from build123d import *

# Parameters (mm, degrees)
SKETCH1_R           = 27.5
BOSS_EXTRUDE1_DEPTH = 12


with BuildPart() as part:
    # Sketch1 → Boss-Extrude1 (new body)
    with BuildSketch(Plane.XY):
        Circle(SKETCH1_R)
        with BuildLine():
            Line((-3.977272727, 12.900825619), (-3.977272727, 17.042045114))
            ThreePointArc((-3.977272727, 17.042045114), (0, 17.5), (3.977272727, 17.042045114))
            Line((3.977272727, 17.042045114), (3.977272727, 12.900825619))
            ThreePointArc((3.977272727, 12.900825619), (6.75, 11.691342951), (9.183806352, 9.894832029))
            Line((9.183806352, 9.894832029), (12.770207637, 11.965441776))
            ThreePointArc((12.770207637, 11.965441776), (15.155444566, 8.75), (16.747480364, 5.076603337))
            Line((16.747480364, 5.076603337), (13.16107908, 3.00599359))
            ThreePointArc((13.16107908, 3.00599359), (13.5, 0), (13.16107908, -3.00599359))
            Line((13.16107908, -3.00599359), (16.747480364, -5.076603337))
            ThreePointArc((16.747480364, -5.076603337), (15.155444566, -8.75), (12.770207637, -11.965441776))
            Line((12.770207637, -11.965441776), (9.183806352, -9.894832029))
            ThreePointArc((9.183806352, -9.894832029), (6.75, -11.691342951), (3.977272727, -12.900825619))
            Line((3.977272727, -12.900825619), (3.977272727, -17.042045114))
            ThreePointArc((3.977272727, -17.042045114), (0, -17.5), (-3.977272727, -17.042045114))
            Line((-3.977272727, -17.042045114), (-3.977272727, -12.900825619))
            ThreePointArc((-3.977272727, -12.900825619), (-6.75, -11.691342951), (-9.183806352, -9.894832029))
            Line((-9.183806352, -9.894832029), (-12.770207637, -11.965441776))
            ThreePointArc((-12.770207637, -11.965441776), (-15.155444566, -8.75), (-16.747480364, -5.076603337))
            Line((-16.747480364, -5.076603337), (-13.16107908, -3.00599359))
            ThreePointArc((-13.16107908, -3.00599359), (-13.5, 0), (-13.16107908, 3.00599359))
            Line((-13.16107908, 3.00599359), (-16.747480364, 5.076603337))
            ThreePointArc((-16.747480364, 5.076603337), (-15.155444566, 8.75), (-12.770207637, 11.965441776))
            Line((-12.770207637, 11.965441776), (-9.183806352, 9.894832029))
            ThreePointArc((-9.183806352, 9.894832029), (-6.75, 11.691342951), (-3.977272727, 12.900825619))
        make_face(mode=Mode.SUBTRACT)
    extrude(amount=BOSS_EXTRUDE1_DEPTH)


solid = part.part
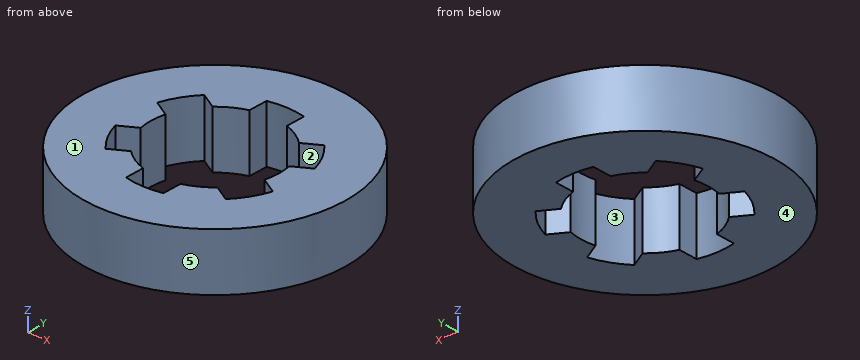
Geometry check sheet. Reference: the model listing, model coordinates, mm. Face numbers are marked on the shaded views. A direction names the side the tool comes from. Coordinates: 2 decimals unless noted, no trailing zeros. Order: outer loops, then holes, each group sorted by start corner. A loop starts at its lowest first (then second) coordinate and runs counter-clockwise, first axis right, second up. Notation, with made-up numbers: (-24, 28.5) -> (7, 28.5) arc R20 cw to (7, 64.5) -> close; hole circle Ø4 at (22, -38). An arc over 180 degrees is marked (long way). Use a Markdown table: item, result. Add a question column.
1. Go/stop test with flat-tipped pins: pin 1 Ø5 at (y, z) = (3.5, 8.5) entering from +X; pin 2 Ø2 at (y, z) = (14, 6) entering from -X; pin 3 Ø1.5 at (x, z) = (-12, 5.5) entering from -Y. Record where each tip stops, or that it passes through.
2. Mould release check, pull along X, two halves, no side actions. Record for the marked faces 3, 4 and 5: pulls with the +X half, pulls with the -X half, needs draft (parallel to the pull), parting line crosses it, or undercut.
3. Material ranges on L1, parallel to X at y = 9, z = 3.25; L2, parallel to X at y = 6, z = 11; L3, parallel to X at y = 11.5, z = 2, recorded low to high.
4. Cross-section at B-B (y = 0). Enter the section's corners in (x, z).
5. Cross-section at A-A (x = 0). Enter the section's corners in (y, z), and give its area (3 significant figures).
6. Cross-section at C-C (z = 8.75). Enter the section's corners in (x, y).
7. Cross-section at D-D (x = 15). Enter the section's corners in (y, z).
8. Set-up check for the marked faces 1 and 2: record each of +Z, -Z, +X, -X, +Y, -Y from which the full face is reachable in a straight line by a thin tool's end or side.
Filled sheet:
| question | item | result |
|---|---|---|
| 1 | pin 1 | x = 27.48 |
| 1 | pin 2 | x = -24.23 |
| 1 | pin 3 | y = -25.09 |
| 2 | face 3 | undercut |
| 2 | face 4 | needs draft |
| 2 | face 5 | parting line crosses it |
| 3 | L1 | -25.99 to -15.01, 15.01 to 25.99 |
| 3 | L2 | -26.84 to -16.44, 16.44 to 26.84 |
| 3 | L3 | -24.98 to -13.19, -11.96 to -7.07, 7.07 to 11.96, 13.19 to 24.98 |
| 4 | outline | (-27.5, 0) -> (-13.5, 0) -> (-13.5, 12) -> (-27.5, 12) -> close; (13.5, 0) -> (27.5, 0) -> (27.5, 12) -> (13.5, 12) -> close |
| 5 | outline | (-27.5, 0) -> (-17.5, 0) -> (-17.5, 12) -> (-27.5, 12) -> close; (17.5, 0) -> (27.5, 0) -> (27.5, 12) -> (17.5, 12) -> close |
| 5 | area | 240 mm2 |
| 6 | outline | circle Ø55 at (0, 0); hole (-16.75, -5.08) arc R17.5 ccw to (-12.77, -11.97) -> (-9.18, -9.89) arc R13.5 ccw to (-3.98, -12.9) -> (-3.98, -17.04) arc R17.5 ccw to (3.98, -17.04) -> (3.98, -12.9) arc R13.5 ccw to (9.18, -9.89) -> (12.77, -11.97) arc R17.5 ccw to (16.75, -5.08) -> (13.16, -3.01) arc R13.5 ccw to (13.16, 3.01) -> (16.75, 5.08) arc R17.5 ccw to (12.77, 11.97) -> (9.18, 9.89) arc R13.5 ccw to (3.98, 12.9) -> (3.98, 17.04) arc R17.5 ccw to (-3.98, 17.04) -> (-3.98, 12.9) arc R13.5 ccw to (-9.18, 9.89) -> (-12.77, 11.97) arc R17.5 ccw to (-16.75, 5.08) -> (-13.16, 3.01) arc R13.5 ccw to (-13.16, -3.01) -> close |
| 7 | outline | (-23.05, 0) -> (-9.01, 0) -> (-9.01, 12) -> (-23.05, 12) -> close; (-4.07, 0) -> (4.07, 0) -> (4.07, 12) -> (-4.07, 12) -> close; (9.01, 0) -> (23.05, 0) -> (23.05, 12) -> (9.01, 12) -> close |
| 8 | face 1 | +Z, +X, -X, +Y, -Y |
| 8 | face 2 | +Z, -Z |
